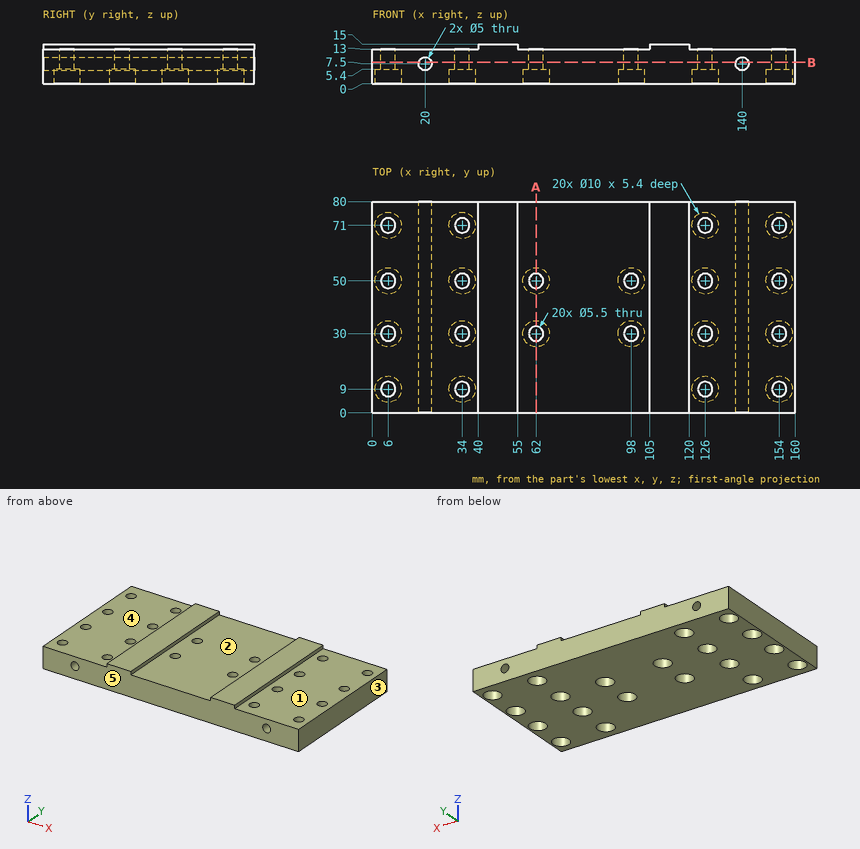
Input: dimensioned drawing with shaded views. Units: mm. Origin: part minimum x, y, z. A direction names the side the tool comes from. Coordinates: 2 decimals unless noted, no trailing zeros. Order: outer loops, then holes, each group sorted by start corner. A loop starts at its lowest first (then second) coordinate and runs counter-clockwise, first axis right, second up. Notation, with made-up numbers: (56.25, -7) -> (112.25, -7) arc R24 ccw to (112.25, 13) -> close; hole circle Ø8 at (-15.5, 52.25). An arc over 180 degrees is marked (long way). Answer in a Markdown table with one row per item.
Item 1: Contact query for flat-ended pins moving along their axis: P1, Ø6, axis at x = 126, y = 71, coming from the -Z side; P2, Ø16, axis at x = 34, y = 50, coming from the -Z side; P3, Ø6, axis at x = 126, y = 9, coming from the +Z side; P4, Ø0.6, axis at y = 58, z = 14, coming from the +X side. Output: stop coordinate, or through.
Return value:
| item | result |
|---|---|
| P1 | stops at z = 5.4 |
| P2 | stops at z = 0 |
| P3 | stops at z = 13 |
| P4 | stops at x = 120 |
Item 2: Section A-A on x = 62. Output: boundary loops of the cut face in (y, z), plus the area to 3 significant figures.
Return value:
| item | result |
|---|---|
| outline | (0, 0) -> (25, 0) -> (25, 5.4) -> (27.25, 5.4) -> (27.25, 13) -> (0, 13) -> close; (32.75, 5.4) -> (35, 5.4) -> (35, 0) -> (45, 0) -> (45, 5.4) -> (47.25, 5.4) -> (47.25, 13) -> (32.75, 13) -> close; (52.75, 5.4) -> (55, 5.4) -> (55, 0) -> (80, 0) -> (80, 13) -> (52.75, 13) -> close |
| area | 848 mm² |
Item 3: Draft query along X for the marked faces 1, 2 and 3. Return one class per face: released by +X, released by -X, zero draft, split by the parting line, or undercut.
Return value:
| item | result |
|---|---|
| face 1 | zero draft |
| face 2 | undercut |
| face 3 | released by +X |
Item 4: Ray query, L1, parallel to Y at x = 98, z = 8; L2, parallel to X at y = 46, z = 14.25; L3, parallel to X at y = 27, z = 7.5. Return the intervals inside material, ascending.
Return value:
| item | result |
|---|---|
| L1 | y = 0 to 27.25, 32.75 to 47.25, 52.75 to 80 |
| L2 | x = 40 to 55, 105 to 120 |
| L3 | x = 0 to 17.5, 22.5 to 137.5, 142.5 to 160 |
Item 5: Access query for the marked faces 4 and 5. Directions: +Z, -Z, +X, -X, +Y, -Y. A direction counts if a zero-diameter tool reaches every point of the face in a straight line with its end or side. Return the directions, or none.
Return value:
| item | result |
|---|---|
| face 4 | +Z, -X, +Y, -Y |
| face 5 | +Z, -Z, +X, -X, -Y |
Item 6: Section B-B on z = 8. State how many separate pieces and enclosed holes the cut face has, plus the area to 3 significant figures.
Return value:
| item | result |
|---|---|
| separate pieces | 3 |
| enclosed holes | 20 |
| area | 11,500 mm² |
